Autodesk Inventor part; units mm, degrees
ref_plane "YZ Plane" through (0, 0, 0) normal (1, 0, 0) x (0, 1, 0)
ref_plane "XZ Plane" through (0, 0, 0) normal (0, 1, 0) x (-1, 0, 0)
ref_plane "XY Plane" through (0, 0, 0) normal (0, 0, 1) x (1, 0, 0)
sketch "スケッチ1" plane through (0, 0, 0) normal (1, 0, 0) x (0, 1, 0)
  circle A0 centre (0, 0) radius 9
  line L0 (9, 0) -> (-9, 0)
  line L1 (-9, 0) -> (-9, 18)
  line L2 (-9, 18) -> (9, 18)
  line L3 (9, 18) -> (9, 0)
  dimension "d0" = 18
  dimension "d1" = 18
  dimension "d2" = 18
extrude "押し出し1" add sketch "スケッチ1" along normal blind 3
sketch "スケッチ2" plane through (3, 0, 0) normal (1, 0, 0) x (0, 0, -1)
  line L0 (-18, 9) -> (-18, -9)
  line L1 (-18, -9) -> (-15, -9)
  line L2 (-15, -9) -> (-15, 9)
  line L3 (-15, 9) -> (-18, 9)
  line L4 (-18, 9) -> (-18, -9)
  line L5 (0, 9) -> (-18, 9)
  point P0 (0, 0)
  dimension "d5" = 3
extrude "押し出し2" add sketch "スケッチ2" along normal blind 38.7
sketch "スケッチ3" plane through (41.7, 0, 0) normal (1, 0, 0) x (0, 0, -1)
  line L0 (-15, 9) -> (-15, -9)
  line L1 (-15, -9) -> (0, -9)
  arc A0 (0, -9) -> (0, 9) centre (0, 0) ccw
  line L2 (0, 9) -> (-15, 9)
  line L3 (-15, -9) -> (-15, 9)
  line L4 (-15, 9) -> (-18, 9)
  line L5 (-18, 9) -> (-18, -9)
  line L6 (-18, -9) -> (-15, -9)
extrude "押し出し3" add sketch "スケッチ3" along normal blind 3
sketch "スケッチ7" plane through (0, -9, 18) normal (0, 0, 1) x (1, 0, 0)
  line L0 (3, 0) -> (41.7, 0)
  line L1 (31.35, 18) -> (13.35, 18)
  line L2 (13.35, 18) -> (13.35, 0)
  line L3 (13.35, 0) -> (31.35, 0)
  line L4 (31.35, 0) -> (31.35, 18)
  line L5 (31.35, 18) -> (13.35, 0) construction
  line L6 (13.35, 18) -> (31.35, 0) construction
  line L7 (0, 18) -> (44.7, 18)
  line L8 (44.7, 18) -> (44.7, 0)
  point P0 (0, 9)
  point P1 (22.35, 9)
  point P2 (31.35, 0)
  dimension "d23" = 18
  dimension "d24" = 22.35
extrude "押し出し7" add sketch "スケッチ7" along normal blind 100
sketch "スケッチ8" plane through (44.7, 0, 0) normal (1, 0, 0) x (0, 0, -1)
  circle A0 centre (0, 0) radius 6 construction
  line L0 (7.1439, 0) -> (-7.1439, 0) construction
  point P0 (-6, 0)
  point P1 (-4.2426, -4.2426)
  point P2 (0, -6)
  point P3 (4.2426, -4.2426)
  point P4 (6, 0)
  point P5 (4.2426, 4.2426)
  point P6 (0, 6)
  point P7 (-4.2426, 4.2426)
  dimension "d27" = 12
  dimension "d30" = 360
hole "穴1" at (44.7, 0, 6) at (44.7, -4.2426, 4.2426) at (44.7, -6, 0) at (44.7, -4.2426, -4.2426) at (44.7, 0, -6) at (44.7, 4.2426, -4.2426) at (44.7, 6, 0) at (44.7, 4.2426, 4.2426) direction (-1, 0, 0) diameter 2.4 depth 6.3
sketch "スケッチ9" plane through (3, 0, 0) normal (1, 0, 0) x (0, 0, -1)
  circle A0 centre (0, 0) radius 3
  dimension "d39" = 6
extrude "押し出し8" add sketch "スケッチ9" along normal blind 5
chamfer "面取り1" distance 5 angle 45 2 edges at (3, 0, 15) (41.7, 0, 15)
chamfer "面取り2" distance 3 angle 45 2 edges at (0, 0, 18) (44.7, 0, 18)
properties part number "Arm2"
Could you check a few things on this model? Use its own coordinates, in mm. A direction names the side the tool comes from. Round coordinates to 2 decimals unless told otherwise and drop trailing zeros. Loops run counter-clockwise (first coordinate to the right, second up) from the corner with the lowest first, then second, coordinate; pieces in that order, holes last. Notation, with made-up numbers: (-37.5, -29) -> (20.5, -29) arc R20 ccw to (20.5, -10) -> close; hole circle Ø2 at (59, 79.5). An arc over 180 degrees is marked (long way). One line per question, with ' | ' between items.
(1) If I drill on probe 1 along X at (y, z) = (0.75, 8.5); probe 2 along Y at (x, z) = (44, 6); probe 3 along X at (y, z) = (8, 35), over which ranges is the centre line in solid material (lowest first)?
Model answer:
probe 1: x = 0 to 3, 41.7 to 44.7 | probe 2: y = -9 to -1.2, 1.2 to 9 | probe 3: x = 13.35 to 31.35
(2) If we section it at C-C on z = 22.5: List the corners of the cut face in (x, y) for me, and give its area (3 significant figures).
Model answer:
outline: (13.35, -9) -> (31.35, -9) -> (31.35, 9) -> (13.35, 9) -> close | area: 324 mm^2
(3) For pin 1 Ø1 at (y, z) = (4.5, 82) entering from +X; pin 2 Ø1.4 at (y, z) = (0, 6) entering from +X; pin 3 Ø3 at (x, y) = (26, 3.5) entering from -Z, each with a flat end and sliding along its axis, tell me the tip position at first contact or that it passes through.
Model answer:
pin 1: stops at x = 31.35 | pin 2: stops at x = 3 | pin 3: stops at z = 15
(4) If we section it at B-B on x = 33: List the corners of the cut face in (y, z) for me, and give its area (3 significant figures).
Model answer:
outline: (-9, 15) -> (9, 15) -> (9, 18) -> (-9, 18) -> close | area: 54.0 mm^2
(5) For faces 4 (the face through (22, 9, 59)), 5 (the face through (8, 0, 18)), 6 (the face through (5, 0, 3)), 7 (the face through (39.2, 0.1, 12.5)), 8 (the face through (43.18, 5.31, 3.69)), which set-ups out of +Z, -Z, +X, -X, +Y, -Y let a thin tool reach every point of the face, with its end or its side?
Model answer:
face 4: +Z, -Z, +X, -X, +Y | face 5: +Z, -X, +Y, -Y | face 6: none | face 7: -Z, +Y, -Y | face 8: +X
(6) If we section it at A-A on y = 0: List the corners of the cut face in (x, z) for me, and give its area (3 significant figures).
Model answer:
outline: (0, -9) -> (3, -9) -> (3, -3) -> (8, -3) -> (8, 3) -> (3, 3) -> (3, 10) -> (8, 15) -> (36.7, 15) -> (41.7, 10) -> (41.7, 7.2) -> (44.7, 7.2) -> (44.7, 15) -> (41.7, 18) -> (31.35, 18) -> (31.35, 118) -> (13.35, 118) -> (13.35, 18) -> (3, 18) -> (0, 15) -> close; (41.7, -9) -> (44.7, -9) -> (44.7, -7.2) -> (41.7, -7.2) -> close; (41.7, -4.8) -> (44.7, -4.8) -> (44.7, 4.8) -> (41.7, 4.8) -> close | area: 2,110 mm^2
(7) Thinking about a two-plate mould opening in Z: for faces 1 (the face through (43.18, -7.01, -0.65)), 2 (the face through (22, 0, 15)), 3 (the face through (43.2, 0.1, 16.5)), which applies, released by +Z, released by -Z, zero draft, split by the parting line, or undercut?
Model answer:
face 1: undercut | face 2: released by -Z | face 3: released by +Z
